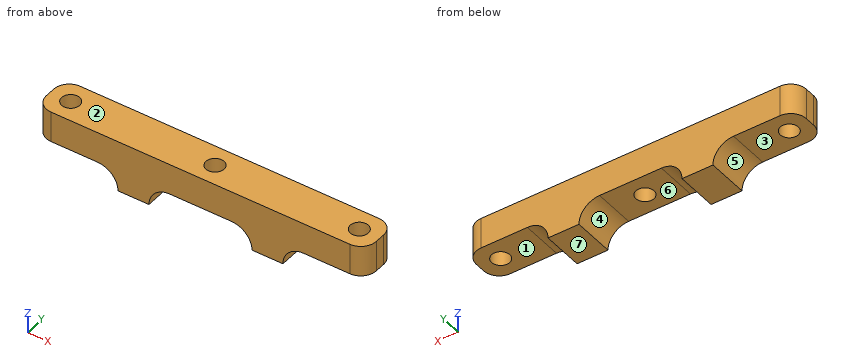
```python
from build123d import *

# Parameters (mm, degrees)
F0_W     = 64
F0_H     = 8
F0_R     = 1.75
F1_DEPTH = 10
F3_DEPTH = 10
F4_R     = 3


with BuildPart() as f1:
    # F0 (on Top) → F1 (new body)
    with BuildSketch(Plane.XY):
        with Locations((32, 4)):
            Rectangle(F0_W, F0_H)
        with Locations((4, 4)):
            Circle(F0_R, mode=Mode.SUBTRACT)
        with Locations((32, 4)):
            Circle(F0_R, mode=Mode.SUBTRACT)
        with Locations((60, 4)):
            Circle(F0_R, mode=Mode.SUBTRACT)
    extrude(amount=F1_DEPTH)

    # F2 (on face) → F3 (cut)
    with BuildSketch(Plane.XZ):
        with BuildLine():
            ThreePointArc((52, 4), (49.171573, 2.828427), (48, 0))
            Line((48, 0), (64, 0))
            Line((64, 0), (64, 4))
            Line((64, 4), (52, 4))
        make_face()
        with BuildLine():
            ThreePointArc((26, 4), (23.171573, 2.828427), (22, 0))
            Line((22, 0), (42, 0))
            ThreePointArc((42, 0), (40.828427, 2.828427), (38, 4))
            Line((38, 4), (26, 4))
        make_face()
        with BuildLine():
            ThreePointArc((16, 0), (14.828427, 2.828427), (12, 4))
            Line((12, 4), (0, 4))
            Line((0, 4), (0, 0))
            Line((0, 0), (16, 0))
        make_face()
    extrude(amount=-F3_DEPTH, mode=Mode.SUBTRACT)

    # F4
    f4_edges = [f1.edges().sort_by_distance(p)[0] for p in [
        (0, 0, 7),
        (0, 8, 7),
        (64, 0, 7),
        (64, 8, 7),
    ]]
    fillet(f4_edges, radius=F4_R)


solid = f1.part
```
The listing builds one solid part. Answer for the finished solid, in the listing's coordinates (mm). Face numbers are marked on the shaded views. A direction names the side the tool comes from. Coordinates: 2 decimals unless noted, no trailing zeros. Loops run counter-clockwise (first coordinate to the right, second up) from the corner with the lowest first, then second, coordinate; pieces in that order, holes last. Notation, with made-up numbers: (-32.5, 53.5) -> (1.5, 53.5) arc R26 ccw to (1.5, 88.5) -> close; hole circle Ø4 at (21.25, 67). An arc over 180 degrees is marked (long way). Return JSON: item names as keys, results as strings. Group by question number.
(1) Find the intervals of material crossed by probe 1 along X at (y, z) = (4, 7.65); probe 2 along Y at (x, z) = (4, 6.4); probe 3 along Z at (x, y) = (30.5, 2.5), in increasing order. Write a range as from..to.
(2) A cutting plane is placed at C-C on z = 5. Write down the section's boundary in (x, y).
(3) Determine the mould class of the marked faces 4, 5, 6 and 7 for opening direction X: released by +X, released by -X, zero draft, split by the parting line, or undercut.
(4) Given pin 1 Ø1 at (x, z) = (9.5, 2.5) entering from -Y; pin 2 Ø3 at (x, z) = (47, 3) entering from -Y; pin 3 Ø4.5 at (x, y) = (60, 4) entering from -Z; pin 4 Ø1.5 at (y, z) = (5, 2) entering from +X, each flat-ended and moving along its own axis, determine where each tip first touches the part or whether it passes through.
(5) A cutting plane is placed at A-A on y = 4. Write down the section's boundary in (x, z).
(6) A cutting plane is placed at B-B on x = 4. Write down the section's boundary in (y, z), and give its area (3 significant figures).
(7) A cutting plane is placed at D-D on z = 1. Write down the section's boundary in (x, y).
(8) Which of the six approach directions +Z, -Z, +X, -X, +Y, -Y give full straight-line access (tool end or side, diameter ignored) to the marked faces 1, 2 and 3?
The answers:
{
 "1": {"probe 1": "x = 0..2.25, 5.75..30.25, 33.75..58.25, 61.75..64", "probe 2": "y = 0..2.25, 5.75..8", "probe 3": "z = 4..10"},
 "2": {"outline": "(0, 3) arc R3 ccw to (3, 0) -> (61, 0) arc R3 ccw to (64, 3) -> (64, 5) arc R3 ccw to (61, 8) -> (3, 8) arc R3 ccw to (0, 5) -> close; hole circle Ø3.5 at (4, 4); hole circle Ø3.5 at (32, 4); hole circle Ø3.5 at (60, 4)"},
 "3": {"face 4": "undercut", "face 5": "released by -X", "face 6": "undercut", "face 7": "zero draft"},
 "4": {"pin 1": "passes through", "pin 2": "stops at y = 0", "pin 3": "stops at z = 4", "pin 4": "stops at x = 49.1"},
 "5": {"outline": "(0, 4) -> (2.25, 4) -> (2.25, 10) -> (0, 10) -> close; (5.75, 4) -> (12, 4) arc R4 cw to (16, 0) -> (22, 0) arc R4 cw to (26, 4) -> (30.25, 4) -> (30.25, 10) -> (5.75, 10) -> close; (33.75, 4) -> (38, 4) arc R4 cw to (42, 0) -> (48, 0) arc R4 cw to (52, 4) -> (58.25, 4) -> (58.25, 10) -> (33.75, 10) -> close; (61.75, 4) -> (64, 4) -> (64, 10) -> (61.75, 10) -> close"},
 "6": {"outline": "(0, 4) -> (2.25, 4) -> (2.25, 10) -> (0, 10) -> close; (5.75, 4) -> (8, 4) -> (8, 10) -> (5.75, 10) -> close", "area": "27.0 mm^2"},
 "7": {"outline": "(15.87, 0) -> (22.13, 0) -> (22.13, 8) -> (15.87, 8) -> close; (41.87, 0) -> (48.13, 0) -> (48.13, 8) -> (41.87, 8) -> close"},
 "8": {"face 1": "-Z, +X, +Y, -Y", "face 2": "+Z, +X, -X, +Y, -Y", "face 3": "-Z, -X, +Y, -Y"}
}
